Read the model definition and answer for the solid it produces. Units are mm, in the model's axes. Face numbers are marked on the shaded views. A direction names the side the tool comes from. Coordinates: 2 decimals unless noted, no trailing zeros. Write each loop counter-clockwise with the first axis right and the second up, starting at its lowest first coordinate (ties: lowest second). Pieces come first, ordered by that corner, then holes.
from build123d import *

# Parameters (mm, degrees)
BOSS_EXTRUDE1_DEPTH = 65
SKETCH2_R           = 2.1
CUT_EXTRUDE1_DEPTH  = 25
SKETCH3_R           = 4
CUT_EXTRUDE2_DEPTH  = 15


with BuildPart() as part:
    # Sketch1 → Boss-Extrude1 (new body)
    with BuildSketch(Plane(origin=(0, 0, 0), x_dir=(0, 0, -1), z_dir=(1, 0, 0))):
        Polygon((0, 0), (0, 18), (7.56469212, 18), (5, 12.5), (22.56469212, 12.5), (20, 7), (25, 7), (25, 0), align=None)
    extrude(amount=BOSS_EXTRUDE1_DEPTH)

    # Sketch2 → Cut-Extrude1 (cut)
    with BuildSketch(Plane(origin=(0, 0, -25), x_dir=(-1, 0, 0), z_dir=(0, 0, -1))):
        with Locations((-12.5, 3.5)):
            Circle(SKETCH2_R)
        with Locations((-52.5, 3.5)):
            Circle(SKETCH2_R)
    extrude(amount=-CUT_EXTRUDE1_DEPTH, mode=Mode.SUBTRACT)

    # Sketch3 → Cut-Extrude2 (cut)
    with BuildSketch(Plane.XY):
        with Locations((12.5, 3.5)):
            Circle(SKETCH3_R)
        with Locations((52.5, 3.5)):
            Circle(SKETCH3_R)
    extrude(amount=-CUT_EXTRUDE2_DEPTH, mode=Mode.SUBTRACT)


solid = part.part
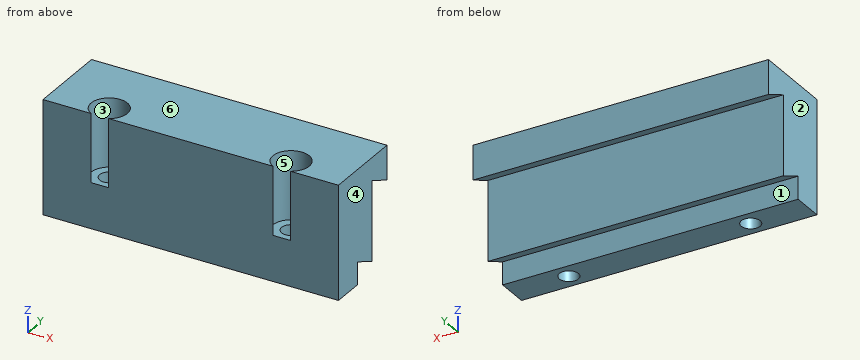
Item 1: The part is cut by section B-B (y = 3.5). Give the vertices of the cut face in (x, z), and give its area (3 significant figures).
Item 2: For the marked faces 1 and 2, determine the directions among +Z, -Z, +X, -X, +Y, -Y from which every point of the face is accessible in a straight line to the end or side of a thin tool.
Item 3: Determine the mould class of the marked faces 3, 4, 5 and 6 for opening direction X: +X half, -X half, draft (parallel to the pull), parting line (faces both ways), or undercut.
Item 4: The part is cut by section A-A (x = 12.5). Give the vertices of the cut face in (y, z).
Item 5: The part is cut by section C-C (z = -18). Give the vertices of the cut face in (x, y), and give its area (3 significant figures).
Item 6: The part is cut by section D-D (x = 46). Give the vertices of the cut face in (y, z), and give its area (3 significant figures).
Item 7: Given pin 1 (1.5 mm diameter, centred on y = 9.5, z = -4, fed in from -X); pin 2 (5 mm diameter, centred on x = 28, z = -21, fed in from +Y); pin 3 (2.5 mm diameter, centred on x = 12.5, y = 3.5, fed in from +Z); pin 4 (7 mm diameter, centred on x = 52.5, y = 3.5, fed in from +Z), each flat-ended and moving along its own axis, determine where each tip first touches the part or whether it passes through.
Item 8: Find the intervals of material crossed by probe 1 along X at (y, z) = (3.5, -9.5); probe 2 along Y at (x, z) = (12.5, -17.5); probe 3 along X at (y, z) = (2.25, -8.25), in increasing order.
Answer:
1. outline: (0, -25) - (10.4, -25) - (10.4, -15) - (8.5, -15) - (8.5, 0) - (0, 0) - close; (14.6, -25) - (50.4, -25) - (50.4, -15) - (48.5, -15) - (48.5, 0) - (16.5, 0) - (16.5, -15) - (14.6, -15) - close; (54.6, -25) - (65, -25) - (65, 0) - (56.5, 0) - (56.5, -15) - (54.6, -15) - close
1. area: 1,300 mm2
2. face 1: -Z, +X, -X
2. face 2: +Z, -Z, -X, +Y, -Y
3. face 3: undercut
3. face 4: +X half
3. face 5: undercut
3. face 6: draft
4. outline: (0, -25) - (1.4, -25) - (1.4, -15) - (0, -15) - close; (5.6, -25) - (7, -25) - (7, -20) - (12.5, -22.56) - (12.5, -5) - (18, -7.56) - (18, 0) - (7.5, 0) - (7.5, -15) - (5.6, -15) - close
5. outline: (0, 0) - (65, 0) - (65, 12.5) - (0, 12.5) - close; hole circle Ø4.2 at (12.5, 3.5); hole circle Ø4.2 at (52.5, 3.5)
5. area: 785 mm2
6. outline: (0, -25) - (7, -25) - (7, -20) - (12.5, -22.56) - (12.5, -5) - (18, -7.56) - (18, 0) - (0, 0) - close
6. area: 327 mm2
7. pin 1: stops at x = 0
7. pin 2: stops at y = 12.5
7. pin 3: passes through
7. pin 4: stops at z = -15
8. probe 1: x = 0 to 8.5, 16.5 to 48.5, 56.5 to 65
8. probe 2: y = 0 to 1.4, 5.6 to 12.5
8. probe 3: x = 0 to 8.7, 16.3 to 48.7, 56.3 to 65
